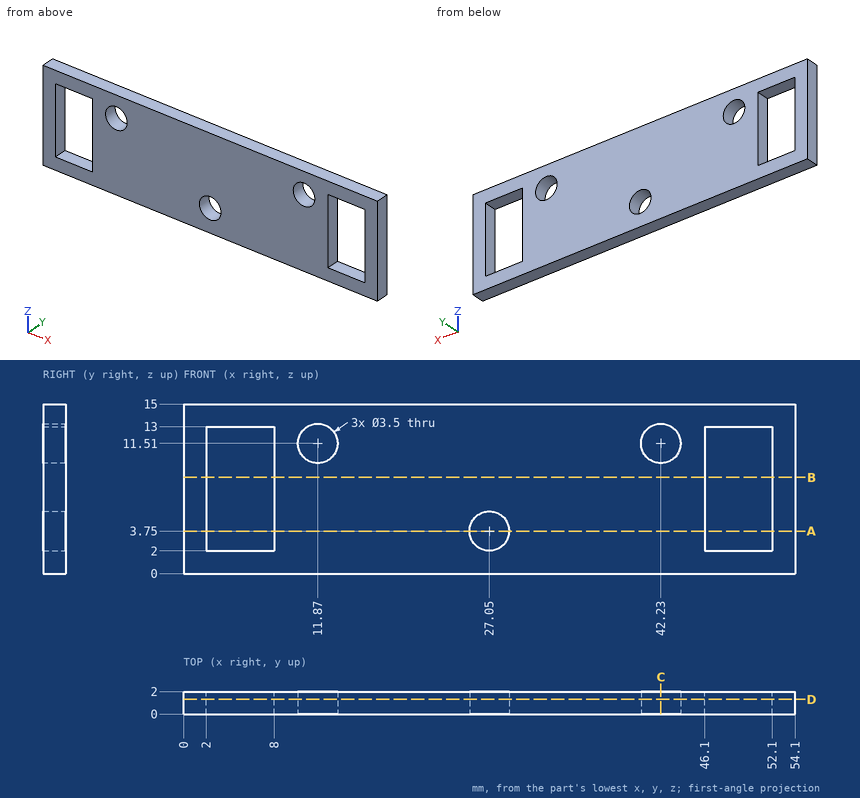
Could you check a few things on this drawing? It's one solid part, dimensions in mm from its lowest x, y, z. Give positions to 0.01 mm unless a question says otherwise; leave off trailing zeros. Order: outer loops, then holes, each group sorted by start corner. A loop starts at its lowest first (then second) coordinate and runs counter-clockwise, first axis right, second up. Notation, with made-up numbers: (61, -2) - (111, -2) arc R24 ccw to (111, 11) - close; hole circle Ø7 at (45, 18.25). An arc over 180 degrees is marked (long way). Answer as a JSON object with one key per item and string values. Group by question number.
Item 1: If we section it at D-D on y = 1.3: Please give me the cut outline in (x, z), and give its area (3 significant figures).
Item 2: For P1, Ø2, axis at x = 27.05, z = 3.75, coming from the -Y side, with a flat end and sliding along its axis, tell me the tip position at first contact or that it passes through.
Item 3: If we section it at A-A on z = 3.75: Please give me the cut outline in (x, y), and give its area (3 significant figures).
Item 4: If we section it at C-C on x = 42.23: Please give me the cut outline in (y, z), and give its area (3 significant figures).
Item 5: If we section it at B-B on z = 8.5: Please give me the cut outline in (x, y).
Item 6: Please list where these lines run through material, in increasing order: probe 1 along X at (y, z) = (1.45, 3.75); probe 2 along X at (y, z) = (1.4, 11.51); probe 3 along X at (y, z) = (1.85, 7).
Result set:
{
 "1": {"outline": "(0, 0) - (54.1, 0) - (54.1, 15) - (0, 15) - close; hole (2, 2) - (8, 2) - (8, 13) - (2, 13) - close; hole circle Ø3.5 at (11.87, 11.51); hole circle Ø3.5 at (27.05, 3.75); hole circle Ø3.5 at (42.23, 11.51); hole (46.1, 2) - (52.1, 2) - (52.1, 13) - (46.1, 13) - close", "area": "651 mm²"},
 "2": {"P1": "through"},
 "3": {"outline": "(0, 0) - (2, 0) - (2, 2) - (0, 2) - close; (8, 0) - (25.3, 0) - (25.3, 2) - (8, 2) - close; (28.8, 0) - (46.1, 0) - (46.1, 2) - (28.8, 2) - close; (52.1, 0) - (54.1, 0) - (54.1, 2) - (52.1, 2) - close", "area": "77.2 mm²"},
 "4": {"outline": "(0, 0) - (2, 0) - (2, 9.76) - (0, 9.76) - close; (0, 13.26) - (2, 13.26) - (2, 15) - (0, 15) - close", "area": "23.0 mm²"},
 "5": {"outline": "(0, 0) - (2, 0) - (2, 2) - (0, 2) - close; (8, 0) - (46.1, 0) - (46.1, 2) - (8, 2) - close; (52.1, 0) - (54.1, 0) - (54.1, 2) - (52.1, 2) - close"},
 "6": {"probe 1": "0 to 2, 8 to 25.3, 28.8 to 46.1, 52.1 to 54.1", "probe 2": "0 to 2, 8 to 10.12, 13.62 to 40.48, 43.98 to 46.1, 52.1 to 54.1", "probe 3": "0 to 2, 8 to 46.1, 52.1 to 54.1"}
}
